CAD build for the part. Positions are in the model's coordinates, mm. Round coordinates to 2 decimals unless told otherwise and drop trailing zeros. Order: outer loops, then holes, each group sorted by start corner. A loop starts at its lowest first (then second) coordinate and runs counter-clockwise, first axis right, second up. Notation, with made-up numbers: (-3.75, 28) - (47.25, 28) arc R10 cw to (47.25, 46) - close; hole circle Ø4 at (72.25, 65). An arc over 180 degrees is marked (long way). Write item = value, one per line.
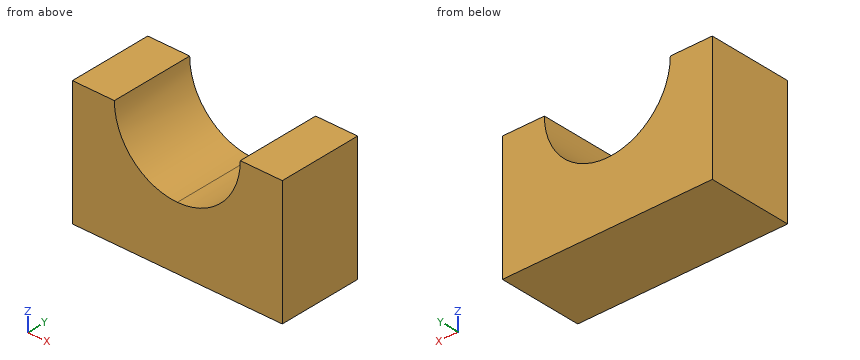
from build123d import *

# Parameters (mm, degrees)
F1_DEPTH = 25.4


with BuildPart() as f1:
    # F0 (on Front) → F1 (new body)
    with BuildSketch(Plane.XZ):
        with BuildLine():
            Line((-62.244336, 47.115693), (-74.944336, 47.115693))
            Line((-74.944336, 47.115693), (-74.944336, 9.015693))
            Line((-74.944336, 9.015693), (-43.194336, 9.015693))
            Line((-43.194336, 9.015693), (-43.194336, 28.065693))
            ThreePointArc((-43.194336, 28.065693), (-56.66472, 33.645309), (-62.244336, 47.115693))
        make_face()
        with BuildLine():
            Line((-11.444336, 47.115693), (-24.144336, 47.115693))
            ThreePointArc((-24.144336, 47.115693), (-29.723952, 33.645309), (-43.194336, 28.065693))
            Line((-43.194336, 28.065693), (-43.194336, 9.015693))
            Line((-43.194336, 9.015693), (-11.444336, 9.015693))
            Line((-11.444336, 9.015693), (-11.444336, 47.115693))
        make_face()
    extrude(amount=F1_DEPTH)


solid = f1.part
(1) Band-saw the part on D-D on x = -39. List the corners of the cut face in (y, z).
Solved:
outline = (-25.4, 9.02) - (0, 9.02) - (0, 28.53) - (-25.4, 28.53) - close
(2) Probe line 1 along X through (y, z) = (-18.5, 45); line 2 along X through (y, z) = (-5, 36); line 3 along Z through (x, y) = (-37.5, -6.25). List the from-to ranges inside material, lowest first.
Solved:
line_1 = -74.94 to -62.13, -24.26 to -11.44
line_2 = -74.94 to -58.67, -27.72 to -11.44
line_3 = 9.02 to 28.94
(3) Band-saw the part on C-C on x = -60.5. List the corners of the cut face in (y, z), plus the area to 3 significant figures.
Solved:
outline = (-25.4, 9.02) - (0, 9.02) - (0, 39.15) - (-25.4, 39.15) - close
area = 765 mm²
(4) Band-saw the part on A-A on y = -15.5. List the corners of the cut face in (x, z), plus the area to 3 significant figures.
Solved:
outline = (-74.94, 9.02) - (-11.44, 9.02) - (-11.44, 47.12) - (-24.14, 47.12) arc R19.05 cw to (-43.19, 28.07) arc R19.05 cw to (-62.24, 47.12) - (-74.94, 47.12) - close
area = 1,850 mm²
(5) Band-saw the part on B-B on z = 32.5. List the corners of the cut face in (x, y).
Solved:
outline = (-74.94, -25.4) - (-55.41, -25.4) - (-55.41, 0) - (-74.94, 0) - close; (-30.98, -25.4) - (-11.44, -25.4) - (-11.44, 0) - (-30.98, 0) - close
